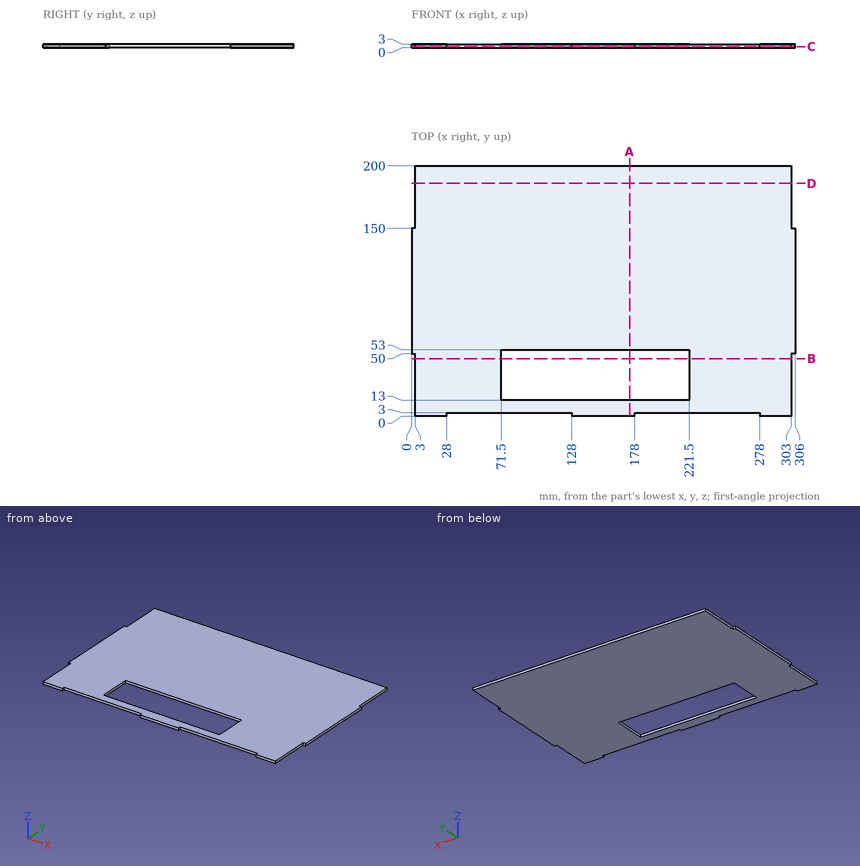
Could you check a few things on this drawing? It's one solid part, dimensions in mm from its lowest x, y, z. Give positions to 0.01 mm unless a question says otherwise; leave off trailing zeros. Loops run counter-clockwise (first coordinate to the right, second up) from the corner with the lowest first, then second, coordinate; pieces in that order, holes last. Notation, with made-up numbers: M 67.5,9 L 98.5,9 A33 cw 98.5,43 Z; hole C 1.5,82 d4. An arc over 180 degrees is marked long. Answer as a JSON object with one key per item and string values.
Q1. For P1, Ø1.5, axis at y = 30, z = 1.5, coming from the -X side; P2, Ø1.5, axis at x = 115, z = 2, coming from the -Y side; P3, Ø8, axis at x = 69, y = 126.5, coming from the -Z side; P4, Ø1.5, axis at x = 305, z = 2, coming from the -Y side, each with a flat end and sliding along its axis, tell me the tip position at first contact or that it passes through.
Values found:
{"P1": "stops at x = 3", "P2": "stops at y = 3", "P3": "stops at z = 0", "P4": "stops at y = 50"}
Q2. If I drill on probe 1 along Y at (x, z) = (125, 0.55); probe 2 along X at (y, z) = (45, 1.25); probe 3 along Y at (x, z) = (132.5, 0.35), over which ranges is the centre line in solid material (lowest first)? Write a range as [from, to].
Values found:
{"probe 1": "y = [3, 13], [53, 200]", "probe 2": "x = [3, 71.5], [221.5, 303]", "probe 3": "y = [0, 13], [53, 200]"}
Q3. Suppose I cut it at A-A, the plane x = 174. List the corners of the cut face in (y, z) for me.
Values found:
{"outline": "M 0,0 L 13,0 L 13,3 L 0,3 Z; M 53,0 L 200,0 L 200,3 L 53,3 Z"}
Q4. Suppose I cut it at D-D, the plane y = 186. List the corners of the cut face in (x, z) for me, plus the area to 3 significant figures.
Values found:
{"outline": "M 3,0 L 303,0 L 303,3 L 3,3 Z", "area": "900 mm²"}
Q5. Suppose I cut it at B-B, the plane y = 46. List the corners of the cut face in (x, z) for me.
Values found:
{"outline": "M 3,0 L 71.5,0 L 71.5,3 L 3,3 Z; M 221.5,0 L 303,0 L 303,3 L 221.5,3 Z"}
Q6. Suppose I cut it at C-C, the plane z = 0.95. List the corners of the cut face in (x, y) for me.
Values found:
{"outline": "M 0,50 L 3,50 L 3,0 L 28,0 L 28,3 L 128,3 L 128,0 L 178,0 L 178,3 L 278,3 L 278,0 L 303,0 L 303,50 L 306,50 L 306,150 L 303,150 L 303,200 L 3,200 L 3,150 L 0,150 Z; hole M 71.5,13 L 221.5,13 L 221.5,53 L 71.5,53 Z"}
